from build123d import *

# Parameters (mm, degrees)
F1_DEPTH = 15.84
F2_DEPTH = 6.21
F3_R     = 1.3


with BuildPart() as f1:
    # F0 (on Top) → F1 (new body)
    with BuildSketch(Plane.XY):
        with BuildLine():
            ThreePointArc((1.985294, -11.073442), (8.628356, -7.219001), (11.25, 0))
            ThreePointArc((11.25, 0), (8.628356, 7.219001), (1.985294, 11.073442))
            ThreePointArc((1.985294, 11.073442), (-11.25, 0), (1.985294, -11.073442))
        make_face()
        with BuildLine():
            ThreePointArc((-5.294396, -1.9), (-5.625, 0), (-5.294396, 1.9))
            ThreePointArc((-5.294396, 1.9), (0, 5.625), (5.294396, 1.9))
            Line((5.294396, 1.9), (7.295, 1.9))
            Line((7.295, 1.9), (7.295, 0))
            Line((7.295, 0), (7.295, -1.9))
            Line((7.295, -1.9), (5.294396, -1.9))
            ThreePointArc((5.294396, -1.9), (0, -5.625), (-5.294396, -1.9))
        make_face(mode=Mode.SUBTRACT)
    extrude(amount=F1_DEPTH)

    # F0 (on Top) → F2 (join)
    with BuildSketch(Plane.XY):
        with BuildLine():
            ThreePointArc((1.985294, 11.073442), (8.628356, 7.219001), (11.25, 0))
            ThreePointArc((11.25, 0), (8.628356, -7.219001), (1.985294, -11.073442))
            Line((1.985294, -11.073442), (22.573529, -7.382294))
            ThreePointArc((22.573529, -7.382294), (28.174792, -2.880495), (27.418746, 4.265744))
            ThreePointArc((27.418746, 4.265744), (25.307311, 6.307791), (22.573529, 7.382294))
            Line((22.573529, 7.382294), (1.985294, 11.073442))
        make_face()
        with BuildLine():
            ThreePointArc((25.25, 0), (17.431624, -1.191639), (24.539998, 2.275063))
            ThreePointArc((24.539998, 2.275063), (25.068376, 1.191639), (25.25, 0))
        make_face(mode=Mode.SUBTRACT)
    extrude(amount=F2_DEPTH)

    # F3
    f3_edges = [f1.edges().sort_by_distance(p)[0] for p in [
        (-1.985294, 11.073442, 15.84),
    ]]
    fillet(f3_edges, radius=F3_R)


solid = f1.part
Design review of the part built by this model. Coordinates are the model's own, in mm. A direction names the side the tool comes from. Round coordinates to 2 decimals unless told otherwise and drop trailing zeros. Loops run counter-clockwise (first coordinate to the right, second up) from the corner with the lowest first, then second, coordinate; pieces in that order, holes last. Notation, with made-up numbers: (60, 2) - (91, 2) arc R4 cw to (91, 7) - close; hole circle Ø5 at (-26, 27.25). An arc over 180 degrees is marked (long way). One line per item, written item: value. Start each with the question number.
1) Consider section B-B on x = 21.25. Give the boundary of the cut face in (y, z), then the cut area to 3 significant figures.
2) To check wall thickness, follow L1, parallel to X at y = 0, z = 4.5 (3 decimals); L2, parallel to Z at x = 26, y = 2.5; L3, parallel to X at y = -0.5, z = 14.75 (3 decimals). State the ranges of each line that lie inside material, in increasing order. Write a range as from..to.
3) For faces 1 (the flat face through (12.135, -9.254, 3.062)), 2 (the flat face through (6, 1.9, 8)), list the 3-axis set-ups (+Z, -Z, +X, -X, +Y, -Y) from which the entire face can be reached by the end or side of a thin tool; tool diameter is ignored.
4) Consider section D-D on y = 1. Give the number of separate pieces and of enclosed holes in the cut face, then the cut area to 3 significant figures.
5) Consider section A-A on z = 8.25. Give the boundary of the cut face in (x, y) (3 decimals), then the cut area to 3 significant figures.
6) Consider section C-C on z = 3. Give the boundary of the cut face in (x, y) (3 decimals).
7) Draft analysis for pull direction X (two halves, no side actions). For faces 3 (the flat face through (8, 0, 0)), 4 (the flat face through (6, -1.9, 8)), 5 (the flat face through (12.424, 9.202, 3.062)), state which applies: +X half, -X half, draft (parallel to the pull), parting line (faces both ways), or undercut.
8) Insertion check: pin 1 Ø1 at (x, y) = (14, 1) entering from -Z; pin 2 Ø4 at (x, z) = (7, 6.5) entering from -Y; pin 3 Ø5 at (y, z) = (4, 2.5) entering from +X; pin 4 Ø3 at (x, y) = (11.5, -4) entering from +Z. Each pin has a flat end and moves straight along its axis. Give the tip position at first contact, or say it passes through.
Reported:
1. outline: (-7.62, 0) - (-4, 0) - (-4, 6.21) - (-7.62, 6.21) - close; (4, 0) - (7.62, 0) - (7.62, 6.21) - (4, 6.21) - close
1. area: 45.0 mm^2
2. L1: x = -11.25..-5.625, 7.295..17.25, 25.25..28.75
2. L2: z = 0..6.21
2. L3: x = -11.222..-5.603, 7.295..11.222
3. face 1: +Z, -Z, +X, -Y
3. face 2: +Z, -Z
4. separate pieces: 3
4. enclosed holes: 0
4. area: 211 mm^2
5. outline: circle Ø22.5 at (0, 0); hole (-5.294, -1.9) arc R5.625 ccw to (5.294, -1.9) - (7.295, -1.9) - (7.295, 1.9) - (5.294, 1.9) arc R5.625 ccw to (-5.294, 1.9) arc R5.625 ccw to start
5. area: 291 mm^2
6. outline: (1.985, -11.073) - (22.574, -7.382) arc R7.5 ccw to (27.419, 4.266) arc R7.5 ccw to (22.574, 7.382) - (1.985, 11.073) arc R11.25 ccw (long way) to start; hole (-5.294, -1.9) arc R5.625 ccw to (5.294, -1.9) - (7.295, -1.9) - (7.295, 1.9) - (5.294, 1.9) arc R5.625 ccw to (-5.294, 1.9) arc R5.625 ccw to start; hole (24.54, 2.275) arc R4 ccw (long way) to (25.25, 0) arc R4 ccw to start
7. face 3: draft
7. face 4: undercut
7. face 5: +X half
8. pin 1: stops at z = 0
8. pin 2: stops at y = -10.53
8. pin 3: stops at x = 28.6
8. pin 4: stops at z = 15.62
